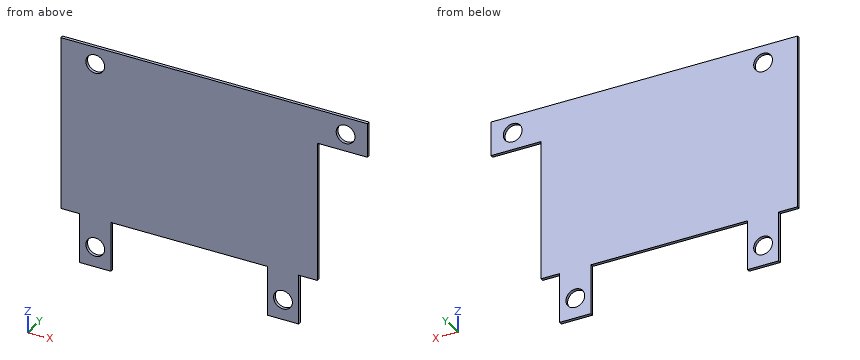
from build123d import *

# Parameters (mm, degrees)
SKETCH1_W           = 41
SKETCH1_H           = 28
BOSS_EXTRUDE1_DEPTH = 0.5
SKETCH2_R           = 1.5
SKETCH2_W           = 5
SKETCH2_H           = 8
SKETCH2_W_2         = 8
SKETCH2_H_2         = 5.5
BOSS_EXTRUDE2_DEPTH = 0.5
SKETCH3_R           = 1.5
CUT_EXTRUDE1_DEPTH  = 1.5


with BuildPart() as part:
    # Sketch1 → Boss-Extrude1 (new body)
    with BuildSketch(Plane(origin=(0, 0, 0), x_dir=(1, 0, 0), z_dir=(0, 1, 0))):
        Rectangle(SKETCH1_W, SKETCH1_H)
    extrude(amount=BOSS_EXTRUDE1_DEPTH)

    # Sketch2 → Boss-Extrude2 (add)
    with BuildSketch(Plane(origin=(0, 0, 0), x_dir=(1, 0, 0), z_dir=(0, 1, 0))):
        with Locations((-15, -11.25)):
            Circle(SKETCH2_R)
        with Locations((-15, 18)):
            Rectangle(SKETCH2_W, SKETCH2_H)
        with Locations((-15, 18.75)):
            Circle(SKETCH2_R, mode=Mode.SUBTRACT)
        with Locations((15, 18)):
            Rectangle(SKETCH2_W, SKETCH2_H)
        with Locations((15, 18.75)):
            Circle(SKETCH2_R, mode=Mode.SUBTRACT)
        with Locations((24.5, -11.25)):
            Rectangle(SKETCH2_W_2, SKETCH2_H_2)
        with Locations((25, -11.25)):
            Circle(SKETCH2_R, mode=Mode.SUBTRACT)
    extrude(amount=BOSS_EXTRUDE2_DEPTH)

    # Sketch3 → Cut-Extrude1 (cut, through all)
    with BuildSketch(Plane(origin=(0, 0.5, 0), x_dir=(1, 0, 0), z_dir=(0, 1, 0))):
        with Locations((-15, -11.25)):
            Circle(SKETCH3_R)
    extrude(amount=-CUT_EXTRUDE1_DEPTH, mode=Mode.SUBTRACT)


solid = part.part
Part model, mm, in its own coordinate system. Coordinates: 2 decimals unless noted, no trailing zeros. Loops run counter-clockwise (first coordinate to the right, second up) from the corner with the lowest first, then second, coordinate; pieces in that order, holes last. Notation, with made-up numbers: (53, 14) -> (102, 14) arc R13 cw to (102, 38) -> close; hole circle Ø6 at (-25, 55.5). An arc over 180 degrees is marked (long way). Use a Markdown table: item, result. Add a question column.
Item 1: Band-saw the part on B-B on x = 15. Write the cut outline in (y, z).
Item 2: Flat gauge pin, fed straight in: P1, Ø1.8, axis at x = 15, z = -18.75, coming from the -Y side. Where does the tip first touch, or does it go through?
Item 3: Band-saw the part on C-C on z = -18.75. Write the cut outline in (x, y), plus the area to 3 significant figures.
Item 4: Band-saw the part on A-A on z = 11.25. Write the cut outline in (x, y), plus the area to 3 significant figures.
Item 5: Probe probe 1 along X at (y, z) = (0.25, 11.25); probe 2 along Z at (x, y) = (-15, 0.25); probe 3 along X at (y, z) = (0.3, -18.75). List the from-to ranges inside material, lowest first.
Item 6: Band-saw the part on D-D on x = -15. Write the cut outline in (y, z), plus the area to 3 significant figures.
Geometry says:
| question | item | result |
|---|---|---|
| 1 | outline | (0, -22) -> (0.5, -22) -> (0.5, -20.25) -> (0, -20.25) -> close; (0, -17.25) -> (0.5, -17.25) -> (0.5, 14) -> (0, 14) -> close |
| 2 | P1 | through |
| 3 | outline | (-17.5, 0) -> (-16.5, 0) -> (-16.5, 0.5) -> (-17.5, 0.5) -> close; (-13.5, 0) -> (-12.5, 0) -> (-12.5, 0.5) -> (-13.5, 0.5) -> close; (12.5, 0) -> (13.5, 0) -> (13.5, 0.5) -> (12.5, 0.5) -> close; (16.5, 0) -> (17.5, 0) -> (17.5, 0.5) -> (16.5, 0.5) -> close |
| 3 | area | 2.00 mm² |
| 4 | outline | (-20.5, 0) -> (-16.5, 0) -> (-16.5, 0.5) -> (-20.5, 0.5) -> close; (-13.5, 0) -> (23.5, 0) -> (23.5, 0.5) -> (-13.5, 0.5) -> close; (26.5, 0) -> (28.5, 0) -> (28.5, 0.5) -> (26.5, 0.5) -> close |
| 4 | area | 21.5 mm² |
| 5 | probe 1 | -20.5 to -16.5, -13.5 to 23.5, 26.5 to 28.5 |
| 5 | probe 2 | -22 to -20.25, -17.25 to 9.75, 12.75 to 14 |
| 5 | probe 3 | -17.5 to -16.5, -13.5 to -12.5, 12.5 to 13.5, 16.5 to 17.5 |
| 6 | outline | (0, -22) -> (0.5, -22) -> (0.5, -20.25) -> (0, -20.25) -> close; (0, -17.25) -> (0.5, -17.25) -> (0.5, 9.75) -> (0, 9.75) -> close; (0, 12.75) -> (0.5, 12.75) -> (0.5, 14) -> (0, 14) -> close |
| 6 | area | 15.0 mm² |
